```python
from build123d import *

# Parameters (mm, degrees)
F0_W     = 8.7125245482
F0_H     = 7.5508523732
F0_R     = 6.8494820219
F0_W_2   = 3.7754308432
F0_H_2   = 7.2604361922
F1_DEPTH = 25.4
F0_W_3   = 6.3891839236
F0_H_3   = 5.5179311894
F0_W_4   = 5.2275173366
F0_H_4   = 7.2604357265
F2_DEPTH = 25.4


with BuildPart() as f1:
    # F0 (on Front) → F1 (new body)
    with BuildSketch(Plane.XZ):
        with Locations((-30.0582041964, 19.7483850643)):
            Rectangle(F0_W, F0_H)
        Polygon((28.6061149091, 23.5238112509), (-25.7019419223, 23.5238112509), (-25.7019419223, 15.9729588777), (-34.4144664705, 15.9729588777), (-34.4144664705, 5.5179311894), (-28.0252825469, 5.5179311894), (-28.0252825469, 0), (27.1540284157, 0), (27.1540284157, 7.2604357265), (32.3815457523, 7.2604357265), (32.3815457523, 16.2633750588), (28.6061149091, 16.2633750588), align=None)
        with Locations((0, 11.3262794912)):
            Circle(F0_R, mode=Mode.SUBTRACT)
        with Locations((30.4938303307, 19.8935931548)):
            Rectangle(F0_W_2, F0_H_2)
    extrude(amount=F1_DEPTH)

    # F0 (on Front) → F2 (join)
    with BuildSketch(Plane.XZ):
        Polygon((-34.4144664705, 15.9729588777), (-34.4144664705, 23.5238112509), (-25.7019419223, 23.5238112509), (-25.7019419223, 27.8800725937), (-38.1898917258, 27.8800725937), (-38.1898917258, 15.9729588777), align=None)
        with Locations((-30.0582041964, 19.7483850643)):
            Rectangle(F0_W, F0_H)
        Polygon((28.6061149091, 23.5238112509), (-25.7019419223, 23.5238112509), (-25.7019419223, 15.9729588777), (-34.4144664705, 15.9729588777), (-34.4144664705, 5.5179311894), (-28.0252825469, 5.5179311894), (-28.0252825469, 0), (27.1540284157, 0), (27.1540284157, 7.2604357265), (32.3815457523, 7.2604357265), (32.3815457523, 16.2633750588), (28.6061149091, 16.2633750588), align=None)
        with Locations((0, 11.3262794912)):
            Circle(F0_R, mode=Mode.SUBTRACT)
        Polygon((28.6061149091, 26.718404144), (28.6061149091, 23.5238112509), (32.3815457523, 23.5238112509), (32.3815457523, 16.2633750588), (38.1898917258, 16.2633750588), (38.1898917258, 26.718404144), align=None)
        with Locations((30.4938303307, 19.8935931548)):
            Rectangle(F0_W_2, F0_H_2)
        with Locations((-31.2198745087, 2.7589655947)):
            Rectangle(F0_W_3, F0_H_3)
        Polygon((-34.4144664705, 0), (-34.4144664705, 5.5179311894), (-39.0611439943, 5.5179311894), (-39.0611439943, -6.0987658799), (-28.0252825469, -6.0987658799), (-28.0252825469, 0), align=None)
        Polygon((37.8994755447, 7.2604357265), (32.3815457523, 7.2604357265), (32.3815457523, 0), (27.1540284157, 0), (27.1540284157, -5.2275136113), (37.8994755447, -5.2275136113), align=None)
        with Locations((29.767787084, 3.6302178632)):
            Rectangle(F0_W_4, F0_H_4)
    extrude(amount=F2_DEPTH)


solid = f1.part
```
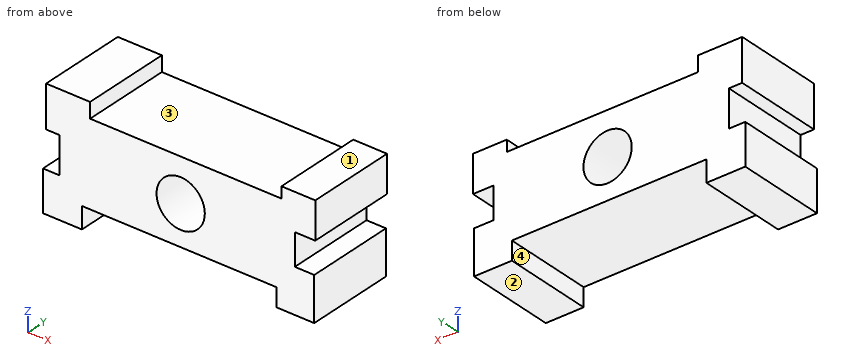
Here's how the part is built. I have some questions about the finished solid (model axes, mm). Face numbers are marked on the shaded views. A direction names the side the tool comes from. Give positions to 0.01 mm unless a question says otherwise; leave off trailing zeros. Loops run counter-clockwise (first coordinate to the right, second up) from the corner with the lowest first, then second, coordinate; pieces in that order, holes last. Notation, with made-up numbers: M 82.5,81 L 135.5,81 A26 ccw 135.5,115 Z; hole C 50,-38.75 d5. An arc over 180 degrees is marked long. Use one line per item in the form item = value. Start each with the question number.
Q1. I need wall thicknesses on line 1 along X through (y, z) = (-13.25, -4); line 2 along Z through (x, y) = (0, -6); line 3 along X through (y, z) = (-21.25, 26). Which ranges of each line are inside material? Lowest first, please.
Q2. If we section it at A-A (z = -4): Write out the boundary of the cut face in (x, y).
Q3. If we section it at D-D (x = -21): Write out the boundary of the cut face in (y, z), then the cut area to 3 significant figures.
Q4. Which directions (+Z, -Z, +X, -X, +Y, -Y) give clear straight access to the entire face, cutting with the end or side of a thin tool? Please do the marked faces 1, 2, 3 and 4.
Q5. If we section it at C-C (y = -10.5): Write out the boundary of the cut face in (x, z).
Q6. If we section it at B-B (x = 0): Write out the boundary of the cut face in (y, z).
Q7. Will these pins go through, and if not, where does the flat tip stop? pin 1 Ø3 at (y, z) = (-10.5, -3) entering from +X; pin 2 Ø1.5 at (y, z) = (-6, 16) entering from -X; pin 3 Ø6 at (x, y) = (-12.5, -10.5) entering from +Z.
Taken from the geometry:
q1.line_1 = -39.06 to -28.03, 27.15 to 37.9
q1.line_2 = 0 to 4.48, 18.18 to 23.52
q1.line_3 = -38.19 to -25.7, 28.61 to 38.19
q2.outline = M -39.06,-25.4 L -28.03,-25.4 L -28.03,0 L -39.06,0 Z; M 27.15,-25.4 L 37.9,-25.4 L 37.9,0 L 27.15,0 Z
q3.outline = M -25.4,0 L 0,0 L 0,23.52 L -25.4,23.52 Z
q3.area = 598 mm^2
q4.face_1 = +Z, +X, +Y, -Y
q4.face_2 = -Z, +X, +Y, -Y
q4.face_3 = +Z, +Y, -Y
q4.face_4 = -Z, +Y, -Y
q5.outline = M -39.06,-6.1 L -28.03,-6.1 L -28.03,0 L 27.15,0 L 27.15,-5.23 L 37.9,-5.23 L 37.9,7.26 L 32.38,7.26 L 32.38,16.26 L 38.19,16.26 L 38.19,26.72 L 28.61,26.72 L 28.61,23.52 L -25.7,23.52 L -25.7,27.88 L -38.19,27.88 L -38.19,15.97 L -34.41,15.97 L -34.41,5.52 L -39.06,5.52 Z; hole C 0,11.33 d13.7
q6.outline = M -25.4,0 L 0,0 L 0,4.48 L -25.4,4.48 Z; M -25.4,18.18 L 0,18.18 L 0,23.52 L -25.4,23.52 Z
q7.pin_1 = 37.9
q7.pin_2 = -38.19
q7.pin_3 = 23.52
